Study the drawing (mm; zero at the part's minimum x, y, z) and answer. A direction names the side the tool comes from. Round coordinates to 2 decimals unless told otherwise and drop trailing zeros. Write each loop counter-clockwise with the first axis right and the second up, starting at its lowest first coordinate (ties: lowest second). Pieces come first, ordered by that corner, then holes.
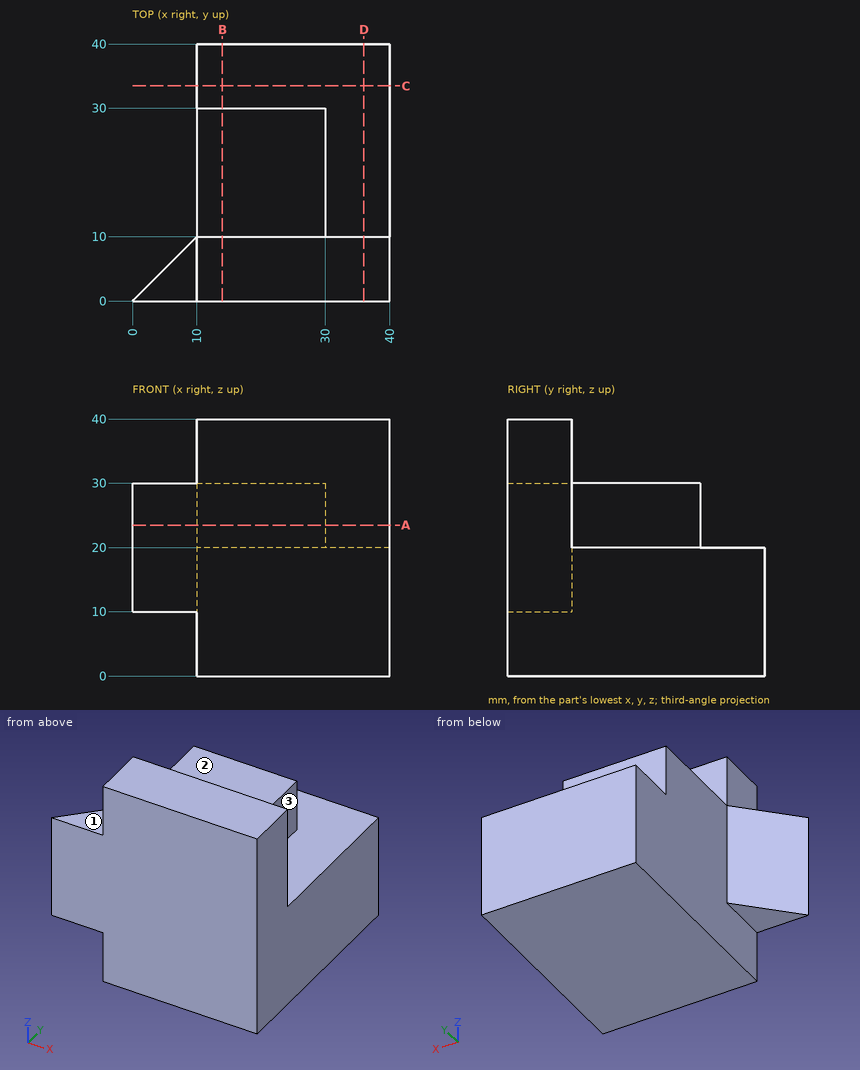
1. Section C-C on y = 33.5 is taken. Determine the outline of the cut face in (x, z).
Geometry says:
outline: (10, 0) - (40, 0) - (40, 20) - (10, 20) - close
2. Section D-D on x = 36 is taken. Determine the outline of the cut face in (y, z), plus the area to 3 significant figures.
Geometry says:
outline: (0, 0) - (40, 0) - (40, 20) - (10, 20) - (10, 40) - (0, 40) - close
area: 1,000 mm2
3. A tool of negligible diameter and unlimited length cuts with its end or side. For the marked faces 1, 2 and 3, from which of +Z, -Z, +X, -X, +Y, -Y can it reach the whole face along a straight path? Write none if from no direction.
Geometry says:
face 1: +Z, -X, +Y, -Y
face 2: +Z, +X, -X, +Y
face 3: +Z, +X, +Y
4. Section A-A on z = 23.5 is taken. Determine the outline of the cut face in (x, y), plus the area to 3 significant figures.
Geometry says:
outline: (0, 0) - (40, 0) - (40, 10) - (30, 10) - (30, 30) - (10, 30) - (10, 10) - close
area: 750 mm2
5. Straight lines are drawn through the part: line 1 along Z through (x, y) = (14, 12); line 2 along Z through (x, y) = (20.5, 37.5); line 3 along X through (y, z) = (11, 5). For each, find the intervals that lie inside material, in ascending order.
Geometry says:
line 1: z = 0 to 30
line 2: z = 0 to 20
line 3: x = 10 to 40
6. Given pin 1 (1 mm diameter, centred on x = 22, y = 15, fed in from +Z); pin 2 (5 mm diameter, centred on x = 25, z = 23, fed in from +Y); pin 3 (12 mm diameter, centred on y = 22.5, z = 31, fed in from +X), each flat-ended and moving along its own axis, determine where each tip first touches the part or whether it passes through.
Geometry says:
pin 1: stops at z = 30
pin 2: stops at y = 30
pin 3: stops at x = 30
7. Section B-B on x = 14 is taken. Determine the outline of the cut face in (y, z).
Geometry says:
outline: (0, 0) - (40, 0) - (40, 20) - (30, 20) - (30, 30) - (10, 30) - (10, 40) - (0, 40) - close
